Can you work these out from the model? Positions are in its coordinate system, mm. A direction names the side the tool comes from. Give positions to 0.01 mm unless a question says otherwise; leave off trailing zeros. Loops run counter-clockwise (first coordinate to the right, second up) from the corner with the lowest first, then second, coordinate; pieces in that order, holes last. Notation, with made-up numbers: (23, 74.5) -> (82, 74.5) arc R21 ccw to (82, 85.5) -> close; hole circle Ø1 at (-15, 1.5). An arc over 180 degrees is marked (long way). One line per question, with ' | ' between items.
from build123d import *

# Parameters (mm, degrees)
SKETCH2_W           = 120
SKETCH2_H           = 120
SKETCH2_R           = 2.5
SKETCH2_W_2         = 87.5
SKETCH2_H_2         = 87.5
BOSS_EXTRUDE1_DEPTH = 5
SKETCH3_W           = 95
SKETCH3_H           = 95
BOSS_EXTRUDE2_DEPTH = 95
CUT_EXTRUDE1_DEPTH  = 95
CUT_EXTRUDE4_REACH  = 191.621
SKETCH5_W           = 87.5
SKETCH5_H           = 87.5
CUT_EXTRUDE5_REACH  = 196.487
SKETCH9_W           = 87.5
SKETCH9_H           = 83.964466094
CUT_EXTRUDE7_DEPTH  = 87.5
BOSS_EXTRUDE3_REACH = 194.683
SKETCH11_W          = 87.5
SKETCH11_H          = 3.75
FILLET1_R           = 10
FILLET2_R           = 5
CUT_EXTRUDE9_DEPTH  = 5.5


with BuildPart() as part:
    # Sketch2 → Boss-Extrude1 (new body)
    with BuildSketch(Plane.XY):
        with Locations((60, -60)):
            Rectangle(SKETCH2_W, SKETCH2_H)
        with Locations((10, -10.00000061)):
            Circle(SKETCH2_R, mode=Mode.SUBTRACT)
        with Locations((110, -10)):
            Circle(SKETCH2_R, mode=Mode.SUBTRACT)
        with Locations((9.988952602, -110)):
            Circle(SKETCH2_R, mode=Mode.SUBTRACT)
        with Locations((109.988952602, -110)):
            Circle(SKETCH2_R, mode=Mode.SUBTRACT)
        with Locations((60, -60)):
            Rectangle(SKETCH2_W_2, SKETCH2_H_2, mode=Mode.SUBTRACT)
    extrude(amount=BOSS_EXTRUDE1_DEPTH)

    # Sketch3 → Boss-Extrude2 (add)
    with BuildSketch(Plane.XY.offset(5)):
        with Locations((60, -60)):
            Rectangle(SKETCH3_W, SKETCH3_H)
    extrude(amount=BOSS_EXTRUDE2_DEPTH)

    # Sketch4 → Cut-Extrude1 (cut)
    with BuildSketch(Plane(origin=(107.5, 0, 0), x_dir=(0, 0, -1), z_dir=(1, 0, 0))):
        Polygon((-5, -12.5), (-100, -107.5), (-100, -12.5), align=None)
    extrude(amount=-CUT_EXTRUDE1_DEPTH, mode=Mode.SUBTRACT)

    # Cut-Extrude4: up to this plane
    cut_extrude4_end = Plane(origin=(12.5, -14.267766953, 3.232233047), z_dir=(0, -0.7071067811865476, -0.7071067811865476))
    # Sketch5 → Cut-Extrude4 (cut, up to the surface)
    with BuildSketch(Plane.XZ.offset(107.5), mode=Mode.PRIVATE) as cut_extrude4_sk1:
        with Locations((60, 52.5)):
            Rectangle(SKETCH5_W, SKETCH5_H)
    cut_extrude4_tool1 = split(extrude(cut_extrude4_sk1.sketch, amount=-CUT_EXTRUDE4_REACH, mode=Mode.PRIVATE), bisect_by=cut_extrude4_end, keep=Keep.BOTH, mode=Mode.PRIVATE)
    add(cut_extrude4_tool1.solids().sort_by_distance((60, -107.5, 52.5))[0], mode=Mode.SUBTRACT)

    # Cut-Extrude5: up to this plane
    cut_extrude5_end = Plane(origin=(12.5, -14.267766953, 3.232233047), z_dir=(0, -0.7071067811865476, -0.7071067811865476))
    # Sketch9 → Cut-Extrude5 (cut, up to the surface)
    with BuildSketch(Plane(origin=(0, 0, 5), x_dir=(-1, 0, 0), z_dir=(0, 0, -1)), mode=Mode.PRIVATE) as cut_extrude5_sk1:
        with Locations((-60, -61.767766953)):
            Rectangle(SKETCH9_W, SKETCH9_H)
    cut_extrude5_tool1 = split(extrude(cut_extrude5_sk1.sketch, amount=-CUT_EXTRUDE5_REACH, mode=Mode.PRIVATE), bisect_by=cut_extrude5_end, keep=Keep.BOTH, mode=Mode.PRIVATE)
    add(cut_extrude5_tool1.solids().sort_by_distance((60, -61.767767, 5))[0], mode=Mode.SUBTRACT)

    # Sketch10 → Cut-Extrude7 (cut)
    with BuildSketch(Plane.ZY.offset(-103.75)):
        Polygon((8.75, -19.785533906), (5, -19.785533906), (5, -16.25), align=None)
    extrude(amount=CUT_EXTRUDE7_DEPTH, mode=Mode.SUBTRACT)

    # Sketch11 → Boss-Extrude3 (add, up to next)
    with BuildSketch(Plane.XY.offset(8.75), mode=Mode.PRIVATE) as boss_extrude3_sk1:
        with Locations((60, -105.625)):
            Rectangle(SKETCH11_W, SKETCH11_H)
    boss_extrude3_tool1 = extrude(boss_extrude3_sk1.sketch, amount=BOSS_EXTRUDE3_REACH, mode=Mode.PRIVATE) - part.part
    add(boss_extrude3_tool1.solids().sort_by_distance((60, -105.625, 8.75))[0])

    # Fillet1
    fillet1_edges = [part.edges().sort_by_distance(p)[0] for p in [
        (0, 0, 2.5),
        (120, 0, 2.5),
        (120, -120, 2.5),
        (0, -120, 2.5),
    ]]
    fillet(fillet1_edges, radius=FILLET1_R)

    # Fillet2
    fillet2_edges = [part.edges().sort_by_distance(p)[0] for p in [
        (12.5, -107.5, 52.5),
        (107.5, -107.5, 52.5),
        (60, -107.5, 100),
        (12.5, -60, 52.5),
        (107.5, -60, 52.5),
    ]]
    fillet(fillet2_edges, radius=FILLET2_R)

    # Sketch16 → Cut-Extrude9 (cut)
    with BuildSketch(Plane.XZ.offset(107.5)):
        with BuildLine():
            Line((20, 82.928932188), (20, 12.5))
            ThreePointArc((20, 12.5), (22.5, 10), (25, 12.5))
            Line((25, 12.5), (25, 82.928932188))
            ThreePointArc((25, 82.928932188), (22.5, 85.428932188), (20, 82.928932188))
        make_face()
        with BuildLine():
            Line((27.5, 82.928932188), (27.5, 12.5))
            ThreePointArc((27.5, 12.5), (30, 10), (32.5, 12.5))
            Line((32.5, 12.5), (32.5, 82.928932188))
            ThreePointArc((32.5, 82.928932188), (30, 85.428932188), (27.5, 82.928932188))
        make_face()
        with BuildLine():
            Line((35, 82.928932188), (35, 12.5))
            ThreePointArc((35, 12.5), (37.5, 10), (40, 12.5))
            Line((40, 12.5), (40, 82.928932188))
            ThreePointArc((40, 82.928932188), (37.5, 85.428932188), (35, 82.928932188))
        make_face()
        with BuildLine():
            Line((42.5, 82.928932188), (42.5, 12.5))
            ThreePointArc((42.5, 12.5), (45, 10), (47.5, 12.5))
            Line((47.5, 12.5), (47.5, 82.928932188))
            ThreePointArc((47.5, 82.928932188), (45, 85.428932188), (42.5, 82.928932188))
        make_face()
        with BuildLine():
            Line((50, 82.928932188), (50, 12.5))
            ThreePointArc((50, 12.5), (52.5, 10), (55, 12.5))
            Line((55, 12.5), (55, 82.928932188))
            ThreePointArc((55, 82.928932188), (52.5, 85.428932188), (50, 82.928932188))
        make_face()
        with BuildLine():
            Line((57.5, 82.928932188), (57.5, 12.5))
            ThreePointArc((57.5, 12.5), (60, 10), (62.5, 12.5))
            Line((62.5, 12.5), (62.5, 82.928932188))
            ThreePointArc((62.5, 82.928932188), (60, 85.428932188), (57.5, 82.928932188))
        make_face()
        with BuildLine():
            Line((65, 82.928932188), (65, 12.5))
            ThreePointArc((65, 12.5), (67.5, 10), (70, 12.5))
            Line((70, 12.5), (70, 82.928932188))
            ThreePointArc((70, 82.928932188), (67.5, 85.428932188), (65, 82.928932188))
        make_face()
        with BuildLine():
            Line((72.5, 82.928932188), (72.5, 12.5))
            ThreePointArc((72.5, 12.5), (75, 10), (77.5, 12.5))
            Line((77.5, 12.5), (77.5, 82.928932188))
            ThreePointArc((77.5, 82.928932188), (75, 85.428932188), (72.5, 82.928932188))
        make_face()
        with BuildLine():
            Line((80, 82.928932188), (80, 12.5))
            ThreePointArc((80, 12.5), (82.5, 10), (85, 12.5))
            Line((85, 12.5), (85, 82.928932188))
            ThreePointArc((85, 82.928932188), (82.5, 85.428932188), (80, 82.928932188))
        make_face()
        with BuildLine():
            Line((87.5, 82.928932188), (87.5, 12.5))
            ThreePointArc((87.5, 12.5), (90, 10), (92.5, 12.5))
            Line((92.5, 12.5), (92.5, 82.928932188))
            ThreePointArc((92.5, 82.928932188), (90, 85.428932188), (87.5, 82.928932188))
        make_face()
        with BuildLine():
            Line((95, 82.928932188), (95, 12.5))
            ThreePointArc((95, 12.5), (97.5, 10), (100, 12.5))
            Line((100, 12.5), (100, 82.928932188))
            ThreePointArc((100, 82.928932188), (97.5, 85.428932188), (95, 82.928932188))
        make_face()
    extrude(amount=-CUT_EXTRUDE9_DEPTH, mode=Mode.SUBTRACT)


solid = part.part
Q1. If we mould it in two halves opening along X, with no side actions, what happens to faces 4 (the face through (12.5, -71, 37)), 5 (the face through (106, -106.07, 47.04)), 6 (the face through (35, -106, 48))? For each: pulls with the +X half, pulls with the -X half, needs draft (parallel to the pull), parting line crosses it, or undercut.
Entries:
face 4: pulls with the -X half | face 5: pulls with the +X half | face 6: undercut
Q2. If I drill on probe 1 along Y at (x, z) = (110, 1.8); probe 2 along Z at (x, y) = (83, -9.5); probe 3 along Y at (x, z) = (72, 85), over which ranges is the centre line in solid material (lowest first)? Write a range as from..to.
Entries:
probe 1: -120..-112.5, -107.5..-12.5, -7.5..0 | probe 2: 0..5 | probe 3: -107.5..-103.75, -96.04..-92.5
Q3. If we section it at B-B (z = 66): State how many separate pieces and enclosed holes the cut face has, plus the area to 3 significant figures.
Entries:
separate pieces: 11 | enclosed holes: 0 | area: 660 mm²
Q4. On a 3-axis mill with a long thin cutter (end or side, diameter ignored), from which of +Z, -Z, +X, -X, +Y, -Y can I reach the whole of each face in a straight line? I mean faces 1 (the face through (107.5, -71, 37)), 2 (the face through (16.25, -70, 35)), 3 (the face through (52.4, -105.7, 10)). Say none if no direction works.
Entries:
face 1: +Z, +X, +Y, -Y | face 2: -Z | face 3: -Y
Q5. For pin 1 Ø12 at (x, y) = (48.5, -66.5) entering from +Z; pin 2 Ø1.1 at (y, z) = (-106, 42) entering from -X; pin 3 Ø10 at (y, z) = (-73.5, 27) entering from -X, each with a flat end and sliding along its axis, tell me the tip position at first contact or that it passes through.
Entries:
pin 1: z = 65 | pin 2: x = 13.46 | pin 3: x = 12.5
Q6. If we section it at C-C (x = 82): Write out the boundary of the cut face in (y, z), plus the area to 3 significant figures.
Entries:
outline: (-120, 0) -> (-103.75, 0) -> (-103.75, 10.05) -> (-107.5, 10.05) -> (-107.5, 5) -> (-120, 5) -> close; (-107.5, 85.38) -> (-103.75, 85.38) -> (-103.75, 92.71) -> (-19.79, 8.75) -> (-16.25, 5) -> (-16.25, 0) -> (0, 0) -> (0, 5) -> (-12.5, 5) -> (-98.96, 91.46) arc R5 ccw to (-107.5, 87.93) -> close | area: 515 mm²
Q7. If we section it at A-A (x = 37.5): Write out the boundary of the cut face in (y, z), plus the area to 3 significant figures.
Entries:
outline: (-120, 0) -> (-103.75, 0) -> (-103.75, 10) -> (-107.5, 10) -> (-107.5, 5) -> (-120, 5) -> close; (-107.5, 85.43) -> (-103.75, 85.43) -> (-103.75, 92.71) -> (-19.79, 8.75) -> (-16.25, 5) -> (-16.25, 0) -> (0, 0) -> (0, 5) -> (-12.5, 5) -> (-98.96, 91.46) arc R5 ccw to (-107.5, 87.93) -> close | area: 515 mm²
